Design review of the part built by this model. Coordinates are the model's own, in mm. Face numbers are marked on the shaded views. Coordinates: 2 decimals unless noted, no trailing zeros. Loops run counter-clockwise (first coordinate to the right, second up) from the corner with the lowest first, then second, coordinate; pieces in that order, holes last. Notation, with made-up numbers: M 9,52 L 24,52 A37 cw 24,89 Z; hole C 88,83 d5. An arc over 180 degrees is marked long. One line per item, written item: value.
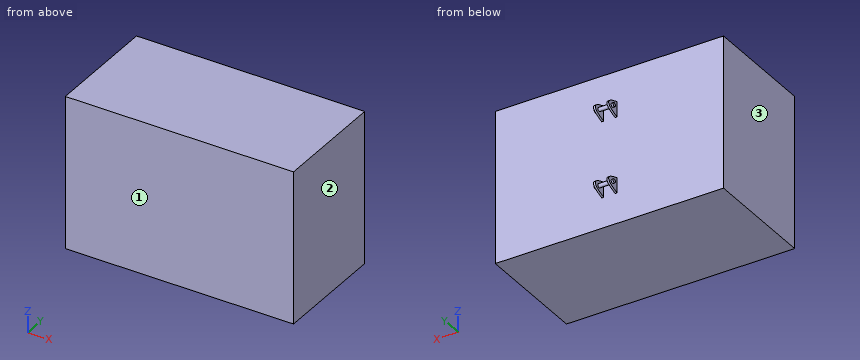
```python
from build123d import *

# Parameters (mm, degrees)
SKETCH2_W                = 400
SKETCH2_H                = 300
BOSS_EXTRUDE1_DEPTH      = 300
BOSS_EXTRUDE1_DEPTH_BACK = 300
BOSS_EXTRUDE4_DEPTH      = 5
BOSS_EXTRUDE5_START      = -20
SKETCH10_R               = 5
BOSS_EXTRUDE5_DEPTH      = 25
MIRROR2_COPY_1_DEPTH     = 5
MIRROR2_START            = -20
MIRROR2_COPY_2_SKETCH_R  = 5
MIRROR2_COPY_2_DEPTH     = 25


with BuildPart() as part:
    # Sketch2 → Boss-Extrude1 (new body, two sides)
    with BuildSketch(Plane(origin=(0, 0, 0), x_dir=(0, 0, -1), z_dir=(1, 0, 0))) as boss_extrude1_sk:
        Rectangle(SKETCH2_W, SKETCH2_H)
    extrude(amount=BOSS_EXTRUDE1_DEPTH)
    extrude(boss_extrude1_sk.sketch, amount=-BOSS_EXTRUDE1_DEPTH_BACK)

    # Sketch9 → Boss-Extrude4 (add)
    with BuildSketch(Plane(origin=(20, 0, 0), x_dir=(0, 0, -1), z_dir=(1, 0, 0))):
        with BuildLine():
            Line((-80, 150), (-100, 150))
            Line((-100, 150), (-120, 150))
            add(Edge.make_bspline(
                [(-120, 150), (-100, 220.369583086), (-80, 150)],
                knots=[0, 0, 0, 1, 1, 1], degree=2))
        make_face()
    boss_extrude4 = extrude(amount=-BOSS_EXTRUDE4_DEPTH)

    # Sketch10 → Boss-Extrude5 (add)
    with BuildSketch(Plane(origin=(20, 0, 0), x_dir=(0, 0, -1), z_dir=(1, 0, 0)).offset(BOSS_EXTRUDE5_START)):
        with Locations((-100.167931578, 169.588362033)):
            Circle(SKETCH10_R)
    boss_extrude5 = extrude(amount=BOSS_EXTRUDE5_DEPTH)

    # Mirror1: Boss-Extrude4, Boss-Extrude5 across plane
    add(boss_extrude4.mirror(Plane(origin=(0, 0, 0), x_dir=(0, 0, 1), z_dir=(1, 0, 0))))
    add(boss_extrude5.mirror(Plane(origin=(0, 0, 0), x_dir=(0, 0, 1), z_dir=(1, 0, 0))))

    # Mirror2: Boss-Extrude5, Boss-Extrude4 across plane
    add(boss_extrude5.mirror(Plane.XY))
    add(boss_extrude4.mirror(Plane.XY))

    # Mirror2 copy 1 sketch → Mirror2 copy 1 (add)
    with BuildSketch(Plane.ZY.offset(20)):
        with BuildLine():
            Line((-80, 150), (-100, 150))
            Line((-100, 150), (-120, 150))
            add(Edge.make_bspline(
                [(-120, 150), (-100, 220.369583086), (-80, 150)],
                knots=[0, 0, 0, 1, 1, 1], degree=2))
        make_face()
    extrude(amount=-MIRROR2_COPY_1_DEPTH)

    # Mirror2 copy 2 sketch → Mirror2 copy 2 (add)
    with BuildSketch(Plane.ZY.offset(20).offset(MIRROR2_START)):
        with Locations((-100.167931578, 169.588362033)):
            Circle(MIRROR2_COPY_2_SKETCH_R)
    extrude(amount=MIRROR2_COPY_2_DEPTH)


solid = part.part
```
(1) We need section B-B on z = -152. State the section outline as (x, y) points, then the cut area to 3 significant figures.
Reply:
outline: M -300,-150 L 300,-150 L 300,150 L -300,150 Z
area: 180,000 mm2
(2) Insertion check: pin 1 (8 mm diameter, centred on y = 168, z = 99.5, fed in from -X); pin 2 (10 mm diameter, centred on x = -171.5, z = -25, fed in from +Y); pin 3 (8 mm diameter, centred on y = 168.5, z = -100, fed in from +X). Each pin has a flat end and moves straight along its axis. Give the tip position at first contact, or say it passes through.
Reply:
pin 1: stops at x = -25
pin 2: stops at y = 150
pin 3: stops at x = 25
(3) To check wall thickness, follow line 1 along Y through (x, z) = (212, -88.5). State the ranges of the line that lie inside material, in increasing order. Write a range as [from, to].
Reply:
line 1: y = [-150, 150]
(4) Mouldability with a two-part tool opening along X and no side actions: class the marked faces 1, 2 and 3 as released by +X, released by -X, zero draft, split by the parting line, or undercut.
Reply:
face 1: zero draft
face 2: released by +X
face 3: released by -X
(5) We need section A-A on x = 111. State the section outline as (y, z) points, then the cut area to 3 significant figures.
Reply:
outline: M -150,-200 L 150,-200 L 150,200 L -150,200 Z
area: 120,000 mm2
